Job drawing, mm, ordinate dimensions from the low corner. One solid piece. A direction names the side the tool comes from. Round coordinates to 2 decimals unless told otherwise and drop trailing zeros. Loops run counter-clockwise (first coordinate to the right, second up) from the corner with the lowest first, then second, coordinate; pieces in that order, holes last.
1) Band-saw the part on A-A, the plane x = 14.5. Write the cut outline in (y, z).
2) Band-saw the part on B-B, the plane y = 8.25. Write the cut outline in (x, z), then the cut area to 3 significant figures.
3) Band-saw the part on C-C, the plane z = 1.51. Write the cut outline in (x, y).
4) Band-saw the part on D-D, the plane x = 47.7. Write the cut outline in (y, z), then the cut area to 3 significant figures.
5) Drop flat-ended pins along their axis: P1, Ø5, axis at y = 2, z = 28, coming from the -X side; P2, Ø6, axis at x = 33.5, z = 14.5, coming from the -Y side; P3, Ø12, axis at x = 51.5, z = 5, coming from the -Y side; P4, Ø1, axis at x = 31.5, y = 5.5, coming from the +Z side. Give the stop position or say it passes through.
6) Probe line 1 (Z direction, x = 53, y = 10.5); line 2 (Z direction, x = 31, y = 1) (1 decimal); line 3 (X direction, y = 7.5, z = 32.5). List the from-to ranges inside material, lowest first.
7) 3-axis set-ups, long thin cutter, end or side, ignore diameter. For the marked faces 1 and 2: which of +Z, -Z, +X, -X, +Y, -Y reach the whole face in a straight line?
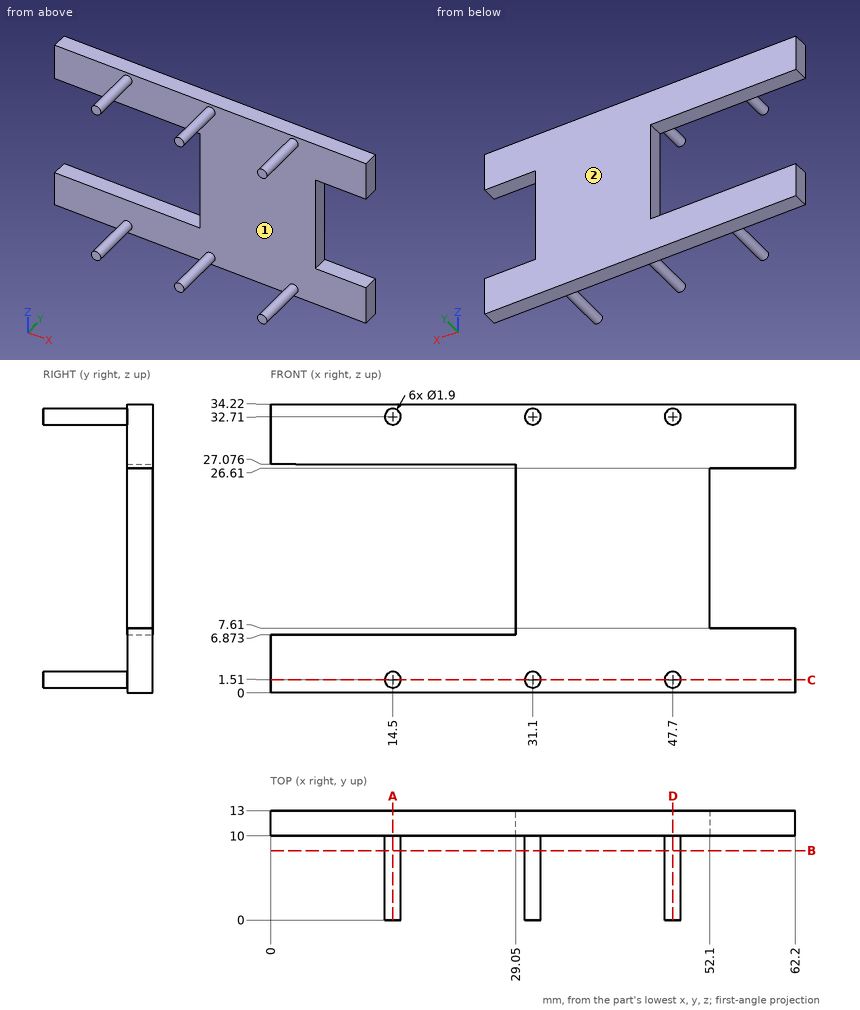
Reported:
1. outline: (0, 0.56) - (10, 0.56) - (10, 0) - (13, 0) - (13, 6.87) - (10, 6.87) - (10, 2.46) - (0, 2.46) - close; (0, 31.76) - (10, 31.76) - (10, 27.08) - (13, 27.08) - (13, 34.22) - (10, 34.22) - (10, 33.66) - (0, 33.66) - close
2. outline: circle Ø1.9 at (14.5, 1.51); circle Ø1.9 at (14.5, 32.71); circle Ø1.9 at (31.1, 1.51); circle Ø1.9 at (31.1, 32.71); circle Ø1.9 at (47.7, 1.51); circle Ø1.9 at (47.7, 32.71)
2. area: 17.0 mm2
3. outline: (0, 10) - (13.55, 10) - (13.55, 0) - (15.45, 0) - (15.45, 10) - (30.15, 10) - (30.15, 0) - (32.05, 0) - (32.05, 10) - (46.75, 10) - (46.75, 0) - (48.65, 0) - (48.65, 10) - (62.2, 10) - (62.2, 13) - (0, 13) - close
4. outline: (0, 0.56) - (10, 0.56) - (10, 0) - (13, 0) - (13, 34.22) - (10, 34.22) - (10, 33.66) - (0, 33.66) - (0, 31.76) - (10, 31.76) - (10, 2.46) - (0, 2.46) - close
4. area: 141 mm2
5. P1: passes through
5. P2: stops at y = 10
5. P3: stops at y = 0
5. P4: stops at z = 33.66
6. line 1: z = 0 to 7.61, 26.61 to 34.22
6. line 2: z = 0.6 to 2.5, 31.8 to 33.7
6. line 3: x = 13.57 to 15.43, 30.17 to 32.03, 46.77 to 48.63
7. face 1: -Y
7. face 2: +Z, -Z, +X, -X, +Y
